Read the model definition and answer for the solid it produces. Units are mm, in the model's axes. Give positions to 0.01 mm unless a question says otherwise; leave off trailing zeros. Loops run counter-clockwise (first coordinate to the right, second up) from the corner with the lowest first, then second, coordinate; pieces in that order, holes last.
(1) Each of these flat-tipped pins is pushed along its axis until it touches: P1, Ø3, axis at x = 0, y = 0, coming from the +Z side; P2, Ø3, axis at x = 2.5, z = 47, coming from the +Y side. Where does it stop, or does it pass through?
(2) Straight lines are drawn through the part: probe 1 along Y at (x, z) = (0, -64.25); probe 2 along Y at (x, z) = (0.25, -51.5); probe 3 along Y at (x, z) = (-0.75, 64). For each, find the intervals that lie inside material, in ascending order.
(3) Find section A-A, the plane z = 9. Write down the section's boundary in (x, y) (1 decimal), then the cut area to 3 significant figures.
(4) Find section B-B, the plane x = 3.5. Write down the section's boundary in (y, z).
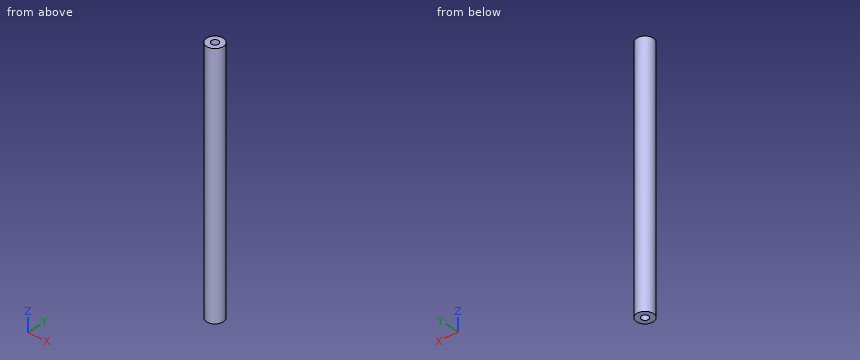
```python
from build123d import *

# Parameters (mm, degrees)
SKETCH1_R                            = 4.7625
BOSS_EXTRUDE1_DEPTH                  = 71.4375
F_10_32_TAPPED_HOLE1_D               = 4.0386
F_10_32_TAPPED_HOLE1_DEPTH           = 11.938
F_10_32_TAPPED_HOLE1_TIP             = 1.213317848
F_10_32_TAPPED_HOLE1_ON_FACE_2_D     = 4.0386
F_10_32_TAPPED_HOLE1_ON_FACE_2_DEPTH = 11.938
F_10_32_TAPPED_HOLE1_ON_FACE_2_TIP   = 1.213317848


with BuildPart() as part:
    # Sketch1 → Boss-Extrude1 (new, symmetric)
    with BuildSketch(Plane.XY):
        Circle(SKETCH1_R)
    extrude(amount=BOSS_EXTRUDE1_DEPTH, both=True)

    # #10-32 Tapped Hole1
    with Locations(Plane.XY.offset(71.4375)):
        with Locations((0, 0)):
            Hole(F_10_32_TAPPED_HOLE1_D / 2, depth=F_10_32_TAPPED_HOLE1_DEPTH)
            with Locations((0, 0, -(F_10_32_TAPPED_HOLE1_DEPTH + F_10_32_TAPPED_HOLE1_TIP / 2))):  # 118° drill point
                Cone(0, F_10_32_TAPPED_HOLE1_D / 2, F_10_32_TAPPED_HOLE1_TIP, mode=Mode.SUBTRACT)

    # #10-32 Tapped Hole1 on face 2
    with Locations(Plane(origin=(0, 0, -71.4375), x_dir=(-1, 0, 0), z_dir=(0, 0, -1))):
        with Locations((0, 0)):
            Hole(F_10_32_TAPPED_HOLE1_ON_FACE_2_D / 2, depth=F_10_32_TAPPED_HOLE1_ON_FACE_2_DEPTH)
            with Locations((0, 0, -(F_10_32_TAPPED_HOLE1_ON_FACE_2_DEPTH + F_10_32_TAPPED_HOLE1_ON_FACE_2_TIP / 2))):  # 118° drill point
                Cone(0, F_10_32_TAPPED_HOLE1_ON_FACE_2_D / 2, F_10_32_TAPPED_HOLE1_ON_FACE_2_TIP, mode=Mode.SUBTRACT)


solid = part.part
```
Entries:
1. P1: stops at z = 59.19
1. P2: stops at y = 4.66
2. probe 1: y = -4.76 to -2.02, 2.02 to 4.76
2. probe 2: y = -4.76 to 4.76
2. probe 3: y = -4.7 to -1.87, 1.87 to 4.7
3. outline: circle Ø9.5 at (0, 0)
3. area: 71.3 mm2
4. outline: (-3.23, -71.44) - (3.23, -71.44) - (3.23, 71.44) - (-3.23, 71.44) - close
